The model under review builds one solid part; all positions refer to its coordinate system, in mm. Round coordinates to 2 decimals unless told otherwise and drop trailing zeros. Loops run counter-clockwise (first coordinate to the right, second up) from the corner with the lowest first, then second, coordinate; pieces in that order, holes last. Notation, with made-up numbers: M 86,-30 L 110,-30 A11 ccw 110,-22 Z; hole C 46.5,-8 d4. An arc over 180 degrees is marked long. One line per question, with ' | ' between items.
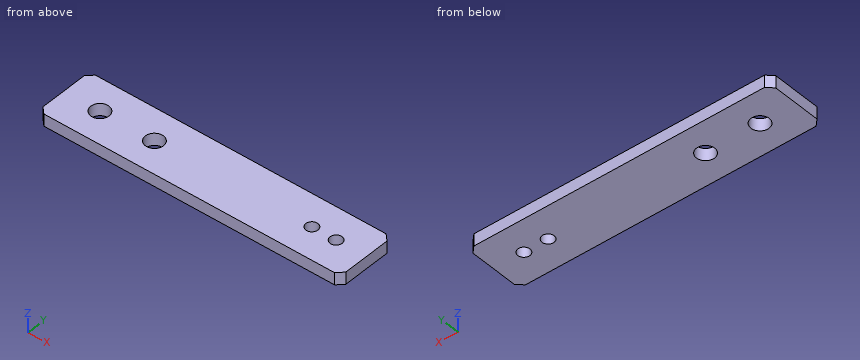
from build123d import *

# Parameters (mm, degrees)
SKETCH1_W           = 50
SKETCH1_H           = 10
SKETCH1_R           = 1.5
SKETCH1_R_2         = 1
BOSS_EXTRUDE1_DEPTH = 2
CHAMFER1_SIZE       = 1


with BuildPart() as part:
    # Sketch1 → Boss-Extrude1 (new body)
    with BuildSketch(Plane.XY):
        with Locations((10.829307568, 4.380032206)):
            Rectangle(SKETCH1_W, SKETCH1_H)
        with Locations((-8.170692432, 4.380032206)):
            Circle(SKETCH1_R, mode=Mode.SUBTRACT)
        with Locations((0.829307568, 4.380032206)):
            Circle(SKETCH1_R, mode=Mode.SUBTRACT)
        with Locations((26.829307568, 4.380032206)):
            Circle(SKETCH1_R_2, mode=Mode.SUBTRACT)
        with Locations((30.829307568, 4.380032206)):
            Circle(SKETCH1_R_2, mode=Mode.SUBTRACT)
    extrude(amount=BOSS_EXTRUDE1_DEPTH)

    # Chamfer1
    chamfer1_edges = [part.edges().sort_by_distance(p)[0] for p in [
        (-14.170692432, 9.380032206, 1),
        (35.829307568, 9.380032206, 1),
        (35.829307568, -0.619967794, 1),
        (-14.170692432, -0.619967794, 1),
    ]]
    chamfer(chamfer1_edges, length=CHAMFER1_SIZE)


solid = part.part
1) Insertion check: P1, Ø2.5, axis at x = -8.17, y = 4.38, coming from the -Z side. The pin has a flat end and moves straight along its axis. Give the tip position at first contact, or say it passes through.
Output values:
P1: passes through
2) Add section B-B on x = 1. State the section outline as (y, z) points, then the cut area to 3 significant figures.
Output values:
outline: M -0.62,0 L 2.89,0 L 2.89,2 L -0.62,2 Z; M 5.87,0 L 9.38,0 L 9.38,2 L 5.87,2 Z | area: 14.0 mm²
3) Add section A-A on z = 1.65. State the section outline as (x, y) points.
Output values:
outline: M -14.17,0.38 L -13.17,-0.62 L 34.83,-0.62 L 35.83,0.38 L 35.83,8.38 L 34.83,9.38 L -13.17,9.38 L -14.17,8.38 Z; hole C -8.17,4.38 d3; hole C 0.83,4.38 d3; hole C 26.83,4.38 d2; hole C 30.83,4.38 d2
4) For line 1 (X direction, y = 4.25, z = 1.7); line 2 (X direction, y = 4.75, z = 1.5); line 3 (X direction, y = 5.5, z = 1.8), list the stretches that pass through material, from the lowest coordinate up.
Output values:
line 1: x = -14.17 to -9.67, -6.68 to -0.67, 2.32 to 25.84, 27.82 to 29.84, 31.82 to 35.83 | line 2: x = -14.17 to -9.62, -6.72 to -0.62, 2.28 to 25.9, 27.76 to 29.9, 31.76 to 35.83 | line 3: x = -14.17 to -9.17, -7.17 to -0.17, 1.83 to 35.83
